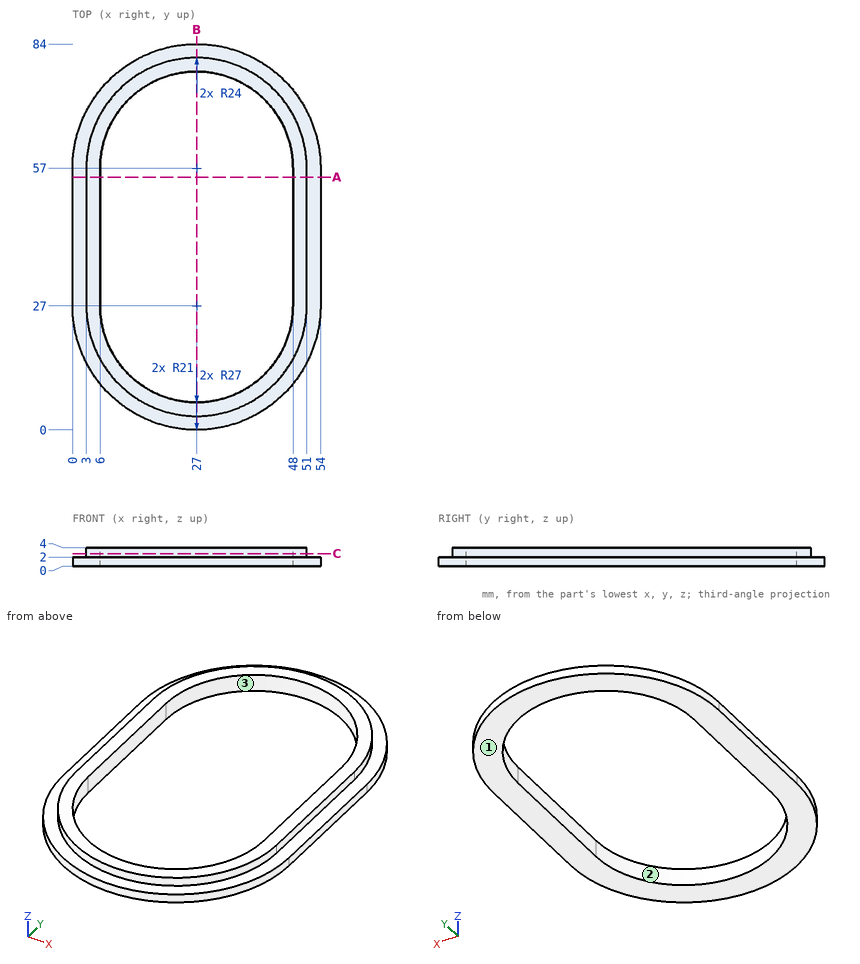
The drawing under review shows one solid part. Ordinate dimensions are in mm from its lowest x, y, z. Coordinates: 2 decimals unless noted, no trailing zeros. Order: outer loops, then holes, each group sorted by start corner. A loop starts at its lowest first (then second) coordinate and runs counter-clockwise, first axis right, second up. Notation, with made-up numbers: (-14, 77) -> (4, 77) arc R19 cw to (4, 98) -> close; hole circle Ø8 at (-12, 53). An arc over 180 degrees is marked (long way). Answer as CSV lines item,"result".
Q1. We need section B-B (x = 27). State the section outline as (y, z) points, plus the area to 3 significant figures.
Model answer:
outline,"(0, 0) -> (6, 0) -> (6, 4) -> (3, 4) -> (3, 2) -> (0, 2) -> close; (78, 0) -> (84, 0) -> (84, 2) -> (81, 2) -> (81, 4) -> (78, 4) -> close"
area,"36.0 mm2"
Q2. Wall thickness on line 1 along X through (y, z) = (34, 0.7); line 2 along X through (y, z) = (57, 2.2); line 3 along Z through (x, y) = (12, 77.5): over which ranges is each line inside the solid? List them lowest first. Write a range as [from, to].
Model answer:
line 1,"x = [0, 6], [48, 54]"
line 2,"x = [3, 6], [48, 51]"
line 3,"z = [0, 2]"
Q3. We need section A-A (y = 55). State the section outline as (x, z) points.
Model answer:
outline,"(0, 0) -> (6, 0) -> (6, 4) -> (3, 4) -> (3, 2) -> (0, 2) -> close; (48, 0) -> (54, 0) -> (54, 2) -> (51, 2) -> (51, 4) -> (48, 4) -> close"
Q4. Clearance check with flat-ended pins moving along their axes: pin 1 Ø0.6 at (y, z) = (36.5, 3) entering from -X; pin 2 Ø5 at (x, y) = (10, 60) entering from -Z. State where each tip first meets the part, or that it passes through.
Model answer:
pin 1,"stops at x = 3"
pin 2,"passes through"
Q5. Draft analysis for pull direction X (two halves, no side actions). For the marked faces 1, 2 and 3, state which applies: released by +X, released by -X, zero draft, split by the parting line, or undercut.
Model answer:
face 1,"zero draft"
face 2,"undercut"
face 3,"undercut"
Q6. We need section C-C (z = 2.75). State the section outline as (x, y) points, plus the area to 3 significant figures.
Model answer:
outline,"(3, 27) arc R24 ccw to (51, 27) -> (51, 57) arc R24 ccw to (3, 57) -> close; hole (6, 27) arc R21 ccw to (48, 27) -> (48, 57) arc R21 ccw to (6, 57) -> close"
area,"604 mm2"
